Geometry check sheet. Reference: the model listing, model coordinates, mm. Face numbers are marked on the shaded views. A direction names the side the tool comes from. Give positions to 0.01 mm unless a question says otherwise; leave off trailing zeros. Order: outer loops, then holes, each group sorted by start corner. A loop starts at its lowest first (then second) coordinate and runs counter-clockwise, first axis right, second up. Notation, with made-up numbers: M 2,27.5 L 43,27.5 A8 cw 43,38.5 Z; hole C -39.75,58.5 d8. An arc over 180 degrees is marked long. Put each result on its own line as item: value. Start each with the question number.
Q1. Section check B-B on y = -10. Record the cut outline in (x, z), then the cut area to 3 significant figures.
Q2. Access from +Z, -Z, +X, -X, +Y, -Y to the whole of each face (thin tool, end or side, straight path). Record for the marked faces 1, 2 and 3.
Q3. Go/stop test with flat-tipped pins: pin 1 (0.9 mm diameter, centred on x = -37.5, y = -71.66, fed in from +Z); pin 2 (1.7 mm diameter, centred on x = -37.5, y = -53.66, fed in from -Z); pin 3 (3 mm diameter, centred on y = -21, z = 5.5, fed in from +X); pin 4 (6 mm diameter, centred on x = -53, y = -11.5, fed in from +Z). Record where each tip stops, or that it passes through.
Q4. Section check A-A on x = -67.5. Record the cut outline in (y, z).
Q5. Section check D-D on y = -29. Record the cut outline in (x, z).
Q6. Material ranges on L1, parallel to Y at x = -67.5, z = 2.5; L2, parallel to Y at x = -37.5, z = 6; L3, parallel to X at y = -12, z = 4, recorded low to high.
Q7. Section check C-C on z = 2.75. Record the cut outline in (x, y), then the cut area to 3 significant figures.
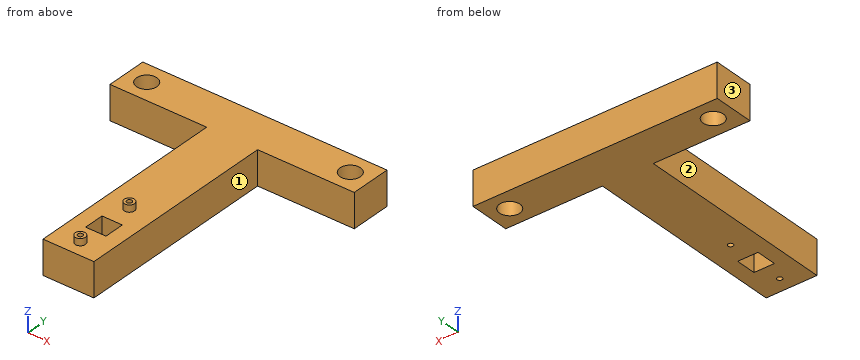
Autodesk Inventor part; units mm, degrees
ref_plane "YZ Plane" through (0, 0, 0) normal (1, 0, 0) x (0, 1, 0)
ref_plane "XZ Plane" through (0, 0, 0) normal (0, 1, 0) x (-1, 0, 0)
ref_plane "XY Plane" through (0, 0, 0) normal (0, 0, 1) x (1, 0, 0)
ref_plane "Płaszczyzna konstrukcyjna1" through (0, -20, 0) normal (0, 0, 1) x (1, 0, 0)
sketch "Szkic1" plane through (0, -20, 0) normal (0, 0, 1) x (1, 0, 0)
  line L0 (-14.5, -19.3841) -> (-60.5, -19.3841) construction
  line L1 (-14.5, -66.5556) -> (-14.5, -19.3841)
  line L2 (-60.5, -66.5556) -> (-14.5, -66.5556)
  line L3 (-60.5, -19.3841) -> (-60.5, -66.5556)
  line L4 (-62.5, -67.9698) -> (-62.5, -17.9698)
  line L5 (-12.5, -67.9698) -> (-62.5, -67.9698)
  line L6 (-12.5, -17.9698) -> (-12.5, -67.9698)
  line L7 (-62.5, -17.9698) -> (-12.5, -17.9698) construction
  circle A0 centre (-7.5, 10) radius 3
  circle A1 centre (-67.5, 10) radius 3
  line L8 (-75, 0) -> (0, 0) construction
  line L9 (0, 20) -> (0, 0)
  line L10 (-75, 20) -> (0, 20)
  line L11 (-75, 20) -> (-75, 0)
  line L12 (-14.5, -19.3841) -> (-60.5, -66.5556) construction
  line L13 (-60.5, -19.3841) -> (-14.5, -66.5556) construction
  line L14 (-1.5, 16) -> (-73.5, 16)
  line L15 (-73.5, 16) -> (-73.5, 4)
  line L16 (-1.5, 4) -> (-1.5, 16)
  line L17 (-27.5, -27.9698) -> (-47.5, -27.9698) construction
  line L18 (-47.5, -27.9698) -> (-47.5, -57.9698) construction
  line L19 (-47.5, -57.9698) -> (-27.5, -57.9698) construction
  line L20 (-27.5, -57.9698) -> (-27.5, -27.9698) construction
  line L21 (-27.5, -27.9698) -> (-47.5, -57.9698) construction
  line L22 (-47.5, -27.9698) -> (-27.5, -57.9698) construction
  line L23 (-37.5, -27.9698) -> (-37.5, -57.9698) construction
  circle A2 centre (-37.5, -33.6556) radius 0.75
  circle A3 centre (-37.5, -51.6556) radius 0.75
  circle A4 centre (-37.5, -33.6556) radius 1.5
  circle A5 centre (-37.5, -51.6556) radius 1.5
  line L24 (-45, 4) -> (-45, -56)
  line L25 (-45, -56) -> (-30, -56)
  line L26 (-30, -56) -> (-30, 4)
  line L27 (-34.5, -39.9698) -> (-40.5, -39.9698)
  line L28 (-40.5, -39.9698) -> (-40.5, -45.9698)
  line L29 (-40.5, -45.9698) -> (-34.5, -45.9698)
  line L30 (-34.5, -45.9698) -> (-34.5, -39.9698)
  line L31 (-34.5, -39.9698) -> (-40.5, -45.9698) construction
  line L32 (-40.5, -39.9698) -> (-34.5, -45.9698) construction
  line L33 (-73.5, 4) -> (-45, 4)
  line L34 (-30, 4) -> (-1.5, 4)
  line L35 (-37.5, -33.6556) -> (-37.5, -51.6556) construction
  point P0 (-37.5, -42.9698)
  point P1 (-1.5, 10)
  point P2 (-37.5, 4)
  dimension "d0" = 6
  dimension "d1" = 6
  dimension "d2" = 6
  dimension "d3" = 20
  dimension "d4" = 30
  dimension "d5" = 1.5
  dimension "d6" = 18
  dimension "d7" = 3
  dimension "d8" = 3
  dimension "d9" = 6
  dimension "d10" = 6
  dimension "d11" = 15
  dimension "d12" = 60
  dimension "d13" = 4.3444
extrude "Wyciągnięcie proste1" add sketch "Szkic1" along normal blind 10 contours L16 L34 L26 L25 L24 L33 L15 L14 | A4 | A5
sketch "Szkic2" plane through (0, -20, 10) normal (0, 0, 1) x (1, 0, 0)
  circle A0 centre (-37.5, -33.6556) radius 1.5
  circle A1 centre (-37.5, -51.6556) radius 1.5
  circle A2 centre (-37.5, -33.6556) radius 0.75
  circle A3 centre (-37.5, -51.6556) radius 0.75
  point P0 (0, 20)
extrude "Wyciągnięcie proste2" add sketch "Szkic2" along normal blind 2
properties part number "camera_holder"
Results found:
1. outline: M -73.5,0 L -70.5,0 L -70.5,10 L -73.5,10 Z; M -64.5,0 L -10.5,0 L -10.5,10 L -64.5,10 Z; M -4.5,0 L -1.5,0 L -1.5,10 L -4.5,10 Z
1. area: 600 mm^2
2. face 1: +Z, -Z, +X, -Y
2. face 2: +Z, -Z, -X, -Y
2. face 3: +Z, -Z, -X, +Y, -Y
3. pin 1: passes through
3. pin 2: stops at z = 0
3. pin 3: stops at x = -30
3. pin 4: stops at z = 10
4. outline: M -16,0 L -13,0 L -13,10 L -16,10 Z; M -7,0 L -4,0 L -4,10 L -7,10 Z
5. outline: M -45,0 L -30,0 L -30,10 L -45,10 Z
6. L1: y = -16 to -13, -7 to -4
6. L2: y = -76 to -72.41, -70.91 to -65.97, -59.97 to -54.41, -52.91 to -4
6. L3: x = -73.5 to -69.74, -65.26 to -9.74, -5.26 to -1.5
7. outline: M -73.5,-16 L -45,-16 L -45,-76 L -30,-76 L -30,-16 L -1.5,-16 L -1.5,-4 L -73.5,-4 Z; hole C -67.5,-10 d6; hole M -40.5,-65.97 L -34.5,-65.97 L -34.5,-59.97 L -40.5,-59.97 Z; hole C -37.5,-71.66 d1.5; hole C -37.5,-53.66 d1.5; hole C -7.5,-10 d6
7. area: 1,670 mm^2
